Source: CAD feature listing. Evaluate the final solid. Frame: model axes, mm. Face numbers are marked on the shaded views. A direction names the side the tool comes from. Give positions to 0.01 mm unless a question says otherwise; leave off trailing zeros. Order: outer loops, then holes, each group sorted by start corner. A loop starts at its lowest first (then second) coordinate and runs counter-clockwise, first axis right, second up. Notation, with made-up numbers: (39.5, 35) -> (65.5, 35) arc R27 cw to (65.5, 56) -> close; hole circle Ø6 at (-21, 46). An arc over 180 degrees is marked (long way). Answer in a Markdown table with one row per item.
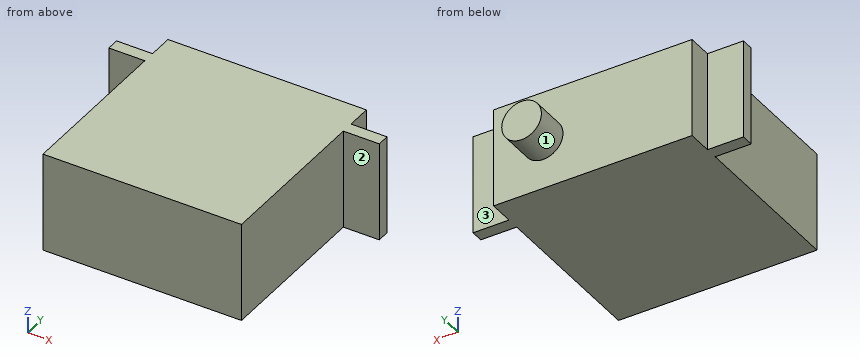
```python
from build123d import *

# Parameters (mm, degrees)
SKETCH1_W           = 40
SKETCH1_H           = 20
BOSS_EXTRUDE1_DEPTH = 40.5
BOSS_EXTRUDE2_START = -5
SKETCH2_W           = 7.25
SKETCH2_H           = 20
BOSS_EXTRUDE2_DEPTH = 2.5
SKETCH3_R           = 10
BOSS_EXTRUDE3_DEPTH = 7
SKETCH4_R           = 10
SKETCH4_R_2         = 4
CUT_EXTRUDE1_DEPTH  = 7


with BuildPart() as part:
    # Sketch1 → Boss-Extrude1 (new body)
    with BuildSketch(Plane(origin=(0, 0, 0), x_dir=(1, 0, 0), z_dir=(0, 1, 0))):
        with Locations((-20, 10)):
            Rectangle(SKETCH1_W, SKETCH1_H)
    extrude(amount=BOSS_EXTRUDE1_DEPTH)

    # Sketch2 → Boss-Extrude2 (add)
    with BuildSketch(Plane(origin=(0, 40.5, 0), x_dir=(1, 0, 0), z_dir=(0, 1, 0)).offset(BOSS_EXTRUDE2_START)):
        with Locations((-43.625, 10)):
            Rectangle(SKETCH2_W, SKETCH2_H)
        with Locations((3.625, 10)):
            Rectangle(SKETCH2_W, SKETCH2_H)
    extrude(amount=-BOSS_EXTRUDE2_DEPTH)

    # Sketch3 → Boss-Extrude3 (add)
    with BuildSketch(Plane(origin=(0, 40.5, 0), x_dir=(1, 0, 0), z_dir=(0, 1, 0))):
        with Locations((-10, 10)):
            Circle(SKETCH3_R)
    extrude(amount=BOSS_EXTRUDE3_DEPTH)

    # Sketch4 → Cut-Extrude1 (cut)
    with BuildSketch(Plane(origin=(0, 47.5, 0), x_dir=(1, 0, 0), z_dir=(0, 1, 0))):
        with Locations((-10, 10)):
            Circle(SKETCH4_R)
        with Locations((-10, 10)):
            Circle(SKETCH4_R_2, mode=Mode.SUBTRACT)
    extrude(amount=-CUT_EXTRUDE1_DEPTH, mode=Mode.SUBTRACT)


solid = part.part
```
(1) Section query B-B (x = -10). Return the cut outline in (y, z).
A:
| item | result |
|---|---|
| outline | (0, -20) -> (40.5, -20) -> (40.5, -14) -> (47.5, -14) -> (47.5, -6) -> (40.5, -6) -> (40.5, 0) -> (0, 0) -> close |
(2) Section query A-A (z = -15.25). Return the cut outline in (x, y), plus the area to 3 significant figures.
A:
| item | result |
|---|---|
| outline | (-47.25, 33) -> (-40, 33) -> (-40, 0) -> (0, 0) -> (0, 33) -> (7.25, 33) -> (7.25, 35.5) -> (0, 35.5) -> (0, 40.5) -> (-40, 40.5) -> (-40, 35.5) -> (-47.25, 35.5) -> close |
| area | 1,660 mm^2 |
(3) Section query D-D (z = -10). Return the cut outline in (x, y), plus the area to 3 significant figures.
A:
| item | result |
|---|---|
| outline | (-47.25, 33) -> (-40, 33) -> (-40, 0) -> (0, 0) -> (0, 33) -> (7.25, 33) -> (7.25, 35.5) -> (0, 35.5) -> (0, 40.5) -> (-6, 40.5) -> (-6, 47.5) -> (-14, 47.5) -> (-14, 40.5) -> (-40, 40.5) -> (-40, 35.5) -> (-47.25, 35.5) -> close |
| area | 1,710 mm^2 |
(4) Access query for the marked faces 1, 2 and 3. Directions: +Z, -Z, +X, -X, +Y, -Y. A direction counts if a zero-diameter tool reaches every point of the face in a straight line with its end or side. Return the directions, or none.
A:
| item | result |
|---|---|
| face 1 | +Y |
| face 2 | +Z, -Z, +X, -Y |
| face 3 | +Z, -Z, +X, +Y |
(5) Section query C-C (y = 42). Return the cut outline in (x, z), plus the area to 3 significant figures.
A:
| item | result |
|---|---|
| outline | circle Ø8 at (-10, -10) |
| area | 50.3 mm^2 |
(6) First-contact query: pin 1 Ø6 at (x, z) = (-19, -6.5) entering from +Y; pin 2 Ø4 at (y, z) = (18.5, -13.5) entering from -X; pin 3 Ø8 at (y, z) = (31.5, -11) entering from +X; pin 4 Ø10 at (y, z) = (12, -13) entering from +X. Flat tips, straight axial feed; report the tip coordinate or a pass-through.
A:
| item | result |
|---|---|
| pin 1 | stops at y = 40.5 |
| pin 2 | stops at x = -40 |
| pin 3 | stops at x = 7.25 |
| pin 4 | stops at x = 0 |
(7) Ray query, probe 1 along X at (y, z) = (8, -17.75); probe 2 along Y at (x, z) = (3.5, -16.5); probe 3 along Y at (x, z) = (-13, -15.5). Return the intervals inside material, ascending.
A:
| item | result |
|---|---|
| probe 1 | x = -40 to 0 |
| probe 2 | y = 33 to 35.5 |
| probe 3 | y = 0 to 40.5 |
